Design review of the part built by this model. Coordinates are the model's own, in mm. A direction names the side the tool comes from. Round coordinates to 2 decimals unless told otherwise and drop trailing zeros. Loops run counter-clockwise (first coordinate to the right, second up) from the corner with the lowest first, then second, coordinate; pieces in that order, holes last. Notation, with made-up numbers: (12, 79) - (34, 79) arc R17 cw to (34, 107) - close; hole circle Ø8 at (39.25, -16). An arc over 180 degrees is marked (long way). Return JSON: item names as keys, results as strings. Group by question number.
(1) The part is to be moulded in two halves that separate along X. For faces 1 (the flat face through (8, 38, 0)), 2 (the flat face through (5, 40, 4)), 3 (the cylindrical face through (0, 24, -10)), 4 (the cylindrical face through (1.802, 27.325, 5.723)), say which applies: pulls with the +X half, pulls with the -X half, needs draft (parallel to the pull), parting line crosses it, or undercut.
(2) We need section A-A, the plane z = 0. Write out the cut boundary in (x, y), and give its area (3 significant figures).
(3) We need section C-C, the plane z = 8. Write out the cut boundary in (x, y), and give its area (3 significant figures).
(4) We need section B-B, the plane x = 3. Write out the cut boundary in (y, z).
(5) We need section D-D, the plane y = 9. Write out the cut boundary in (x, z).
(6) For faces 5 (the flat face through (0, 0, -8)), 6 (the flat face through (0, 7, -6)), 7 (the cylindrical face through (-0.6, 39, -8.8)), list the 3-axis set-ups (+Z, -Z, +X, -X, +Y, -Y) from which the entire face can be reached by the end or side of a thin tool; tool diameter is ignored.
(7) Wall thickness on L1, parallel to X at y = 39.25, z = 0; L2, parallel to Z at x = -0.25, y = 35.5; L3, parallel to Z at x = 8, y = 38.7: over which ranges is each line inside the solid? List them lowest first. Write a range as [from, to].
(8) Clearance check with flat-ended pins moving along their axes: pin 1 (1.2 mm diameter, centred on x = 8, z = 0, fed in from -Y); pin 2 (3 mm diameter, centred on x = 5, y = 11.5, fed in from +Z); pin 3 (1.5 mm diameter, centred on x = 2.5, y = 24, fed in from -Z). State where each tip first meets the part, or that it passes through.
from build123d import *

# Parameters (mm, degrees)
SKETCH_1_R               = 10
SKETCH_1_R_2             = 6
EXTRUDE_1_DEPTH          = 40
SKETCH_2_R               = 1
CUT_EXTRUDE_1_DEPTH      = 2
CUT_EXTRUDE_2_DEPTH      = 43.426406871
CUT_EXTRUDE_2_DEPTH_BACK = 43.426406871
SKETCH_3_W               = 12
SKETCH_3_H               = 15


with BuildPart() as part:
    # 草图1 → 凸台-拉伸1 (new body)
    with BuildSketch(Plane(origin=(0, 0, 0), x_dir=(1, 0, 0), z_dir=(0, 1, 0))):
        with Locations(Location((0, 0, 0), (0, 0, 270))):
            Circle(SKETCH_1_R)
        with Locations(Location((0, 0, 0), (0, 0, 270))):
            Circle(SKETCH_1_R_2, mode=Mode.SUBTRACT)
    extrude(amount=EXTRUDE_1_DEPTH)

    # 草图2 → 切除-拉伸1 (cut)
    with BuildSketch(Plane(origin=(0, 40, 0), x_dir=(1, 0, 0), z_dir=(0, 1, 0))):
        with Locations(Location((-8, 0, 0), (0, 0, 270))):
            Circle(SKETCH_2_R)
        with Locations(Location((8, 0, 0), (0, 0, 90))):
            Circle(SKETCH_2_R)
        with Locations(Location((0, 8, 0), (0, 0, 270))):
            Circle(SKETCH_2_R)
        with Locations(Location((0, -8, 0), (0, 0, 90))):
            Circle(SKETCH_2_R)
    extrude(amount=-CUT_EXTRUDE_1_DEPTH, mode=Mode.SUBTRACT)

    # 草图3 → 切除-拉伸2 (cut, two sides: drawn at the far end of the back side and taken through both)
    with BuildSketch(Plane(origin=(0, 0, 0), x_dir=(0, 0, -1), z_dir=(1, 0, 0)).offset(-CUT_EXTRUDE_2_DEPTH_BACK)):
        with Locations((0, 7.5)):
            Rectangle(SKETCH_3_W, SKETCH_3_H)
    extrude(amount=CUT_EXTRUDE_2_DEPTH + CUT_EXTRUDE_2_DEPTH_BACK, mode=Mode.SUBTRACT)


solid = part.part
Solutions:
{
 "1": {"face 1": "undercut", "face 2": "needs draft", "face 3": "parting line crosses it", "face 4": "undercut"},
 "2": {"outline": "(-10, 15) - (-6, 15) - (-6, 40) - (-7, 40) - (-7, 38) - (-9, 38) - (-9, 40) - (-10, 40) - close; (6, 15) - (10, 15) - (10, 40) - (9, 40) - (9, 38) - (7, 38) - (7, 40) - (6, 40) - close", "area": "192 mm^2"},
 "3": {"outline": "(-6, 0) - (6, 0) - (6, 40) - (1, 40) - (1, 38) - (-1, 38) - (-1, 40) - (-6, 40) - close", "area": "476 mm^2"},
 "4": {"outline": "(0, -9.54) - (40, -9.54) - (40, -5.2) - (15, -5.2) - (15, -6) - (0, -6) - close; (0, 6) - (15, 6) - (15, 5.2) - (40, 5.2) - (40, 9.54) - (0, 9.54) - close"},
 "5": {"outline": "(-8, -6) arc R10 ccw to (8, -6) - close; (-8, 6) - (8, 6) arc R10 ccw to start"},
 "6": {"face 5": "+Z, -Z, +X, -X, -Y", "face 6": "+X, -X, -Y", "face 7": "+Y"},
 "7": {"L1": "[-10, -9], [-7, -6], [6, 7], [9, 10]", "L2": "[-10, -5.99], [5.99, 10]", "L3": "[-6, -1], [1, 6]"},
 "8": {"pin 1": "y = 15", "pin 2": "z = 9.37", "pin 3": "z = -9.85"}
}
